Work out the finished part from the listing and answer in its coordinate system (mm). Round coordinates to 2 decimals unless told otherwise and drop trailing zeros. Loops run counter-clockwise (first coordinate to the right, second up) from the corner with the lowest first, then second, coordinate; pieces in that order, holes last. Notation, with made-up numbers: (34, -39.75) - (92, -39.75) arc R18 ccw to (92, -33.75) - close; hole circle Ø4 at (-26.5, 20.25). An arc over 180 degrees is marked (long way). Return JSON: item names as keys, results as strings.
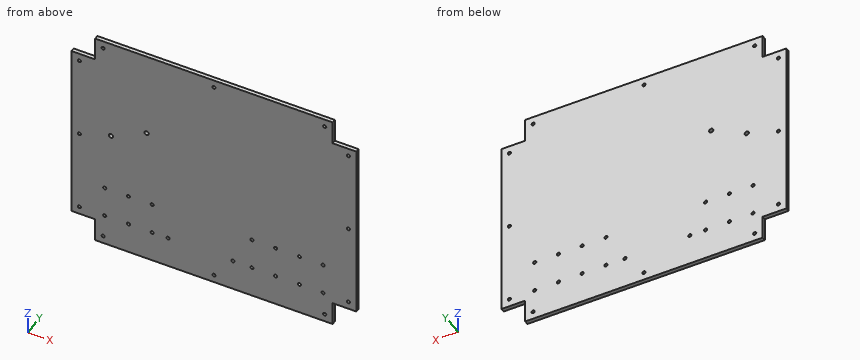
from build123d import *

# Parameters (mm, degrees)
SKETCH1_W           = 457.2
SKETCH1_H           = 368.3
SKETCH1_R           = 2.5527
BOSS_EXTRUDE1_DEPTH = 6.35
CUT_EXTRUDE1_REACH  = 589.126
SKETCH2_W           = 38.1
SKETCH2_H           = 38.1
CUT_EXTRUDE2_REACH  = 589.126
SKETCH3_R           = 2.5527
CUT_EXTRUDE3_REACH  = 589.126
SKETCH5_R           = 3.429


with BuildPart() as part:
    # Sketch1 → Boss-Extrude1 (new body)
    with BuildSketch(Plane(origin=(0, 0, 0), x_dir=(1, 0, 0), z_dir=(0, 1, 0))):
        with Locations((228.6, 184.15)):
            Rectangle(SKETCH1_W, SKETCH1_H)
        with Locations(Location((50.8, 355.6, 0), (0, 0, 270))):
            Circle(SKETCH1_R, mode=Mode.SUBTRACT)
        with Locations(Location((406.4, 355.6, 0), (0, 0, 270))):
            Circle(SKETCH1_R, mode=Mode.SUBTRACT)
        with Locations(Location((406.4, 12.7, 0), (0, 0, 270))):
            Circle(SKETCH1_R, mode=Mode.SUBTRACT)
        with Locations(Location((50.8, 12.7, 0), (0, 0, 270))):
            Circle(SKETCH1_R, mode=Mode.SUBTRACT)
        with Locations(Location((228.6, 12.7, 0), (0, 0, 270))):
            Circle(SKETCH1_R, mode=Mode.SUBTRACT)
        with Locations(Location((228.6, 355.6, 0), (0, 0, 270))):
            Circle(SKETCH1_R, mode=Mode.SUBTRACT)
        with Locations(Location((12.7, 184.15, 0), (0, 0, 270))):
            Circle(SKETCH1_R, mode=Mode.SUBTRACT)
        with Locations(Location((444.5, 184.15, 0), (0, 0, 270))):
            Circle(SKETCH1_R, mode=Mode.SUBTRACT)
        with Locations(Location((12.7, 50.8, 0), (0, 0, 270))):
            Circle(SKETCH1_R, mode=Mode.SUBTRACT)
        with Locations(Location((444.5, 50.8, 0), (0, 0, 270))):
            Circle(SKETCH1_R, mode=Mode.SUBTRACT)
        with Locations(Location((444.5, 317.5, 0), (0, 0, 270))):
            Circle(SKETCH1_R, mode=Mode.SUBTRACT)
        with Locations(Location((12.7, 317.5, 0), (0, 0, 270))):
            Circle(SKETCH1_R, mode=Mode.SUBTRACT)
    extrude(amount=BOSS_EXTRUDE1_DEPTH)

    # Sketch2 → Cut-Extrude1 (cut, up to next)
    with BuildSketch(Plane(origin=(0, 6.35, 0), x_dir=(1, 0, 0), z_dir=(0, 1, 0)), mode=Mode.PRIVATE) as cut_extrude1_sk1:
        with Locations((19.05, 19.05)):
            Rectangle(SKETCH2_W, SKETCH2_H)
    cut_extrude1_tool1 = extrude(cut_extrude1_sk1.sketch, amount=-CUT_EXTRUDE1_REACH, mode=Mode.PRIVATE) & part.part
    # Sketch2 → Cut-Extrude1 (cut, up to next)
    with BuildSketch(Plane(origin=(0, 6.35, 0), x_dir=(1, 0, 0), z_dir=(0, 1, 0)), mode=Mode.PRIVATE) as cut_extrude1_sk2:
        with Locations((19.05, 349.25)):
            Rectangle(SKETCH2_W, SKETCH2_H)
    cut_extrude1_tool2 = extrude(cut_extrude1_sk2.sketch, amount=-CUT_EXTRUDE1_REACH, mode=Mode.PRIVATE) & part.part
    # Sketch2 → Cut-Extrude1 (cut, up to next)
    with BuildSketch(Plane(origin=(0, 6.35, 0), x_dir=(1, 0, 0), z_dir=(0, 1, 0)), mode=Mode.PRIVATE) as cut_extrude1_sk3:
        with Locations((438.15, 349.25)):
            Rectangle(SKETCH2_W, SKETCH2_H)
    cut_extrude1_tool3 = extrude(cut_extrude1_sk3.sketch, amount=-CUT_EXTRUDE1_REACH, mode=Mode.PRIVATE) & part.part
    # Sketch2 → Cut-Extrude1 (cut, up to next)
    with BuildSketch(Plane(origin=(0, 6.35, 0), x_dir=(1, 0, 0), z_dir=(0, 1, 0)), mode=Mode.PRIVATE) as cut_extrude1_sk4:
        with Locations((438.15, 19.05)):
            Rectangle(SKETCH2_W, SKETCH2_H)
    cut_extrude1_tool4 = extrude(cut_extrude1_sk4.sketch, amount=-CUT_EXTRUDE1_REACH, mode=Mode.PRIVATE) & part.part
    add(cut_extrude1_tool1.solids().sort_by_distance((19.05, 6.35, -19.05))[0], mode=Mode.SUBTRACT)
    add(cut_extrude1_tool2.solids().sort_by_distance((19.05, 6.35, -349.25))[0], mode=Mode.SUBTRACT)
    add(cut_extrude1_tool3.solids().sort_by_distance((438.15, 6.35, -349.25))[0], mode=Mode.SUBTRACT)
    add(cut_extrude1_tool4.solids().sort_by_distance((438.15, 6.35, -19.05))[0], mode=Mode.SUBTRACT)

    # Sketch3 → Cut-Extrude2 (cut, up to next)
    with BuildSketch(Plane(origin=(0, 6.35, 0), x_dir=(1, 0, 0), z_dir=(0, 1, 0)), mode=Mode.PRIVATE) as cut_extrude2_sk1:
        with Locations(Location((53.34, 266.7, 0), (0, 0, 270))):
            Circle(SKETCH3_R)
    cut_extrude2_tool1 = extrude(cut_extrude2_sk1.sketch, amount=-CUT_EXTRUDE2_REACH, mode=Mode.PRIVATE) & part.part
    # Sketch3 → Cut-Extrude2 (cut, up to next)
    with BuildSketch(Plane(origin=(0, 6.35, 0), x_dir=(1, 0, 0), z_dir=(0, 1, 0)), mode=Mode.PRIVATE) as cut_extrude2_sk2:
        with Locations(Location((53.34, 317.5, 0), (0, 0, 270))):
            Circle(SKETCH3_R)
    cut_extrude2_tool2 = extrude(cut_extrude2_sk2.sketch, amount=-CUT_EXTRUDE2_REACH, mode=Mode.PRIVATE) & part.part
    # Sketch3 → Cut-Extrude2 (cut, up to next)
    with BuildSketch(Plane(origin=(0, 6.35, 0), x_dir=(1, 0, 0), z_dir=(0, 1, 0)), mode=Mode.PRIVATE) as cut_extrude2_sk3:
        with Locations(Location((91.44, 266.7, 0), (0, 0, 270))):
            Circle(SKETCH3_R)
    cut_extrude2_tool3 = extrude(cut_extrude2_sk3.sketch, amount=-CUT_EXTRUDE2_REACH, mode=Mode.PRIVATE) & part.part
    # Sketch3 → Cut-Extrude2 (cut, up to next)
    with BuildSketch(Plane(origin=(0, 6.35, 0), x_dir=(1, 0, 0), z_dir=(0, 1, 0)), mode=Mode.PRIVATE) as cut_extrude2_sk4:
        with Locations(Location((91.44, 317.5, 0), (0, 0, 270))):
            Circle(SKETCH3_R)
    cut_extrude2_tool4 = extrude(cut_extrude2_sk4.sketch, amount=-CUT_EXTRUDE2_REACH, mode=Mode.PRIVATE) & part.part
    # Sketch3 → Cut-Extrude2 (cut, up to next)
    with BuildSketch(Plane(origin=(0, 6.35, 0), x_dir=(1, 0, 0), z_dir=(0, 1, 0)), mode=Mode.PRIVATE) as cut_extrude2_sk5:
        with Locations(Location((129.54, 266.7, 0), (0, 0, 270))):
            Circle(SKETCH3_R)
    cut_extrude2_tool5 = extrude(cut_extrude2_sk5.sketch, amount=-CUT_EXTRUDE2_REACH, mode=Mode.PRIVATE) & part.part
    # Sketch3 → Cut-Extrude2 (cut, up to next)
    with BuildSketch(Plane(origin=(0, 6.35, 0), x_dir=(1, 0, 0), z_dir=(0, 1, 0)), mode=Mode.PRIVATE) as cut_extrude2_sk6:
        with Locations(Location((129.54, 317.5, 0), (0, 0, 270))):
            Circle(SKETCH3_R)
    cut_extrude2_tool6 = extrude(cut_extrude2_sk6.sketch, amount=-CUT_EXTRUDE2_REACH, mode=Mode.PRIVATE) & part.part
    # Sketch3 → Cut-Extrude2 (cut, up to next)
    with BuildSketch(Plane(origin=(0, 6.35, 0), x_dir=(1, 0, 0), z_dir=(0, 1, 0)), mode=Mode.PRIVATE) as cut_extrude2_sk7:
        with Locations(Location((289.56, 266.7, 0), (0, 0, 270))):
            Circle(SKETCH3_R)
    cut_extrude2_tool7 = extrude(cut_extrude2_sk7.sketch, amount=-CUT_EXTRUDE2_REACH, mode=Mode.PRIVATE) & part.part
    # Sketch3 → Cut-Extrude2 (cut, up to next)
    with BuildSketch(Plane(origin=(0, 6.35, 0), x_dir=(1, 0, 0), z_dir=(0, 1, 0)), mode=Mode.PRIVATE) as cut_extrude2_sk8:
        with Locations(Location((289.56, 317.5, 0), (0, 0, 270))):
            Circle(SKETCH3_R)
    cut_extrude2_tool8 = extrude(cut_extrude2_sk8.sketch, amount=-CUT_EXTRUDE2_REACH, mode=Mode.PRIVATE) & part.part
    # Sketch3 → Cut-Extrude2 (cut, up to next)
    with BuildSketch(Plane(origin=(0, 6.35, 0), x_dir=(1, 0, 0), z_dir=(0, 1, 0)), mode=Mode.PRIVATE) as cut_extrude2_sk9:
        with Locations(Location((403.86, 266.7, 0), (0, 0, 270))):
            Circle(SKETCH3_R)
    cut_extrude2_tool9 = extrude(cut_extrude2_sk9.sketch, amount=-CUT_EXTRUDE2_REACH, mode=Mode.PRIVATE) & part.part
    # Sketch3 → Cut-Extrude2 (cut, up to next)
    with BuildSketch(Plane(origin=(0, 6.35, 0), x_dir=(1, 0, 0), z_dir=(0, 1, 0)), mode=Mode.PRIVATE) as cut_extrude2_sk10:
        with Locations(Location((403.86, 317.5, 0), (0, 0, 270))):
            Circle(SKETCH3_R)
    cut_extrude2_tool10 = extrude(cut_extrude2_sk10.sketch, amount=-CUT_EXTRUDE2_REACH, mode=Mode.PRIVATE) & part.part
    # Sketch3 → Cut-Extrude2 (cut, up to next)
    with BuildSketch(Plane(origin=(0, 6.35, 0), x_dir=(1, 0, 0), z_dir=(0, 1, 0)), mode=Mode.PRIVATE) as cut_extrude2_sk11:
        with Locations(Location((365.76, 266.7, 0), (0, 0, 270))):
            Circle(SKETCH3_R)
    cut_extrude2_tool11 = extrude(cut_extrude2_sk11.sketch, amount=-CUT_EXTRUDE2_REACH, mode=Mode.PRIVATE) & part.part
    # Sketch3 → Cut-Extrude2 (cut, up to next)
    with BuildSketch(Plane(origin=(0, 6.35, 0), x_dir=(1, 0, 0), z_dir=(0, 1, 0)), mode=Mode.PRIVATE) as cut_extrude2_sk12:
        with Locations(Location((365.76, 317.5, 0), (0, 0, 270))):
            Circle(SKETCH3_R)
    cut_extrude2_tool12 = extrude(cut_extrude2_sk12.sketch, amount=-CUT_EXTRUDE2_REACH, mode=Mode.PRIVATE) & part.part
    # Sketch3 → Cut-Extrude2 (cut, up to next)
    with BuildSketch(Plane(origin=(0, 6.35, 0), x_dir=(1, 0, 0), z_dir=(0, 1, 0)), mode=Mode.PRIVATE) as cut_extrude2_sk13:
        with Locations(Location((327.66, 266.7, 0), (0, 0, 270))):
            Circle(SKETCH3_R)
    cut_extrude2_tool13 = extrude(cut_extrude2_sk13.sketch, amount=-CUT_EXTRUDE2_REACH, mode=Mode.PRIVATE) & part.part
    # Sketch3 → Cut-Extrude2 (cut, up to next)
    with BuildSketch(Plane(origin=(0, 6.35, 0), x_dir=(1, 0, 0), z_dir=(0, 1, 0)), mode=Mode.PRIVATE) as cut_extrude2_sk14:
        with Locations(Location((327.66, 317.5, 0), (0, 0, 270))):
            Circle(SKETCH3_R)
    cut_extrude2_tool14 = extrude(cut_extrude2_sk14.sketch, amount=-CUT_EXTRUDE2_REACH, mode=Mode.PRIVATE) & part.part
    # Sketch3 → Cut-Extrude2 (cut, up to next)
    with BuildSketch(Plane(origin=(0, 6.35, 0), x_dir=(1, 0, 0), z_dir=(0, 1, 0)), mode=Mode.PRIVATE) as cut_extrude2_sk15:
        with Locations(Location((259.08, 317.5, 0), (0, 0, 270))):
            Circle(SKETCH3_R)
    cut_extrude2_tool15 = extrude(cut_extrude2_sk15.sketch, amount=-CUT_EXTRUDE2_REACH, mode=Mode.PRIVATE) & part.part
    # Sketch3 → Cut-Extrude2 (cut, up to next)
    with BuildSketch(Plane(origin=(0, 6.35, 0), x_dir=(1, 0, 0), z_dir=(0, 1, 0)), mode=Mode.PRIVATE) as cut_extrude2_sk16:
        with Locations(Location((154.94, 317.5, 0), (0, 0, 270))):
            Circle(SKETCH3_R)
    cut_extrude2_tool16 = extrude(cut_extrude2_sk16.sketch, amount=-CUT_EXTRUDE2_REACH, mode=Mode.PRIVATE) & part.part
    add(cut_extrude2_tool1.solids().sort_by_distance((53.34, 6.35, -266.7))[0], mode=Mode.SUBTRACT)
    add(cut_extrude2_tool2.solids().sort_by_distance((53.34, 6.35, -317.5))[0], mode=Mode.SUBTRACT)
    add(cut_extrude2_tool3.solids().sort_by_distance((91.44, 6.35, -266.7))[0], mode=Mode.SUBTRACT)
    add(cut_extrude2_tool4.solids().sort_by_distance((91.44, 6.35, -317.5))[0], mode=Mode.SUBTRACT)
    add(cut_extrude2_tool5.solids().sort_by_distance((129.54, 6.35, -266.7))[0], mode=Mode.SUBTRACT)
    add(cut_extrude2_tool6.solids().sort_by_distance((129.54, 6.35, -317.5))[0], mode=Mode.SUBTRACT)
    add(cut_extrude2_tool7.solids().sort_by_distance((289.56, 6.35, -266.7))[0], mode=Mode.SUBTRACT)
    add(cut_extrude2_tool8.solids().sort_by_distance((289.56, 6.35, -317.5))[0], mode=Mode.SUBTRACT)
    add(cut_extrude2_tool9.solids().sort_by_distance((403.86, 6.35, -266.7))[0], mode=Mode.SUBTRACT)
    add(cut_extrude2_tool10.solids().sort_by_distance((403.86, 6.35, -317.5))[0], mode=Mode.SUBTRACT)
    add(cut_extrude2_tool11.solids().sort_by_distance((365.76, 6.35, -266.7))[0], mode=Mode.SUBTRACT)
    add(cut_extrude2_tool12.solids().sort_by_distance((365.76, 6.35, -317.5))[0], mode=Mode.SUBTRACT)
    add(cut_extrude2_tool13.solids().sort_by_distance((327.66, 6.35, -266.7))[0], mode=Mode.SUBTRACT)
    add(cut_extrude2_tool14.solids().sort_by_distance((327.66, 6.35, -317.5))[0], mode=Mode.SUBTRACT)
    add(cut_extrude2_tool15.solids().sort_by_distance((259.08, 6.35, -317.5))[0], mode=Mode.SUBTRACT)
    add(cut_extrude2_tool16.solids().sort_by_distance((154.94, 6.35, -317.5))[0], mode=Mode.SUBTRACT)

    # Sketch5 → Cut-Extrude3 (cut, up to next)
    with BuildSketch(Plane.XZ, mode=Mode.PRIVATE) as cut_extrude3_sk1:
        with Locations(Location((63.5, -167.64, 0), (0, 0, 270))):
            Circle(SKETCH5_R)
    cut_extrude3_tool1 = extrude(cut_extrude3_sk1.sketch, amount=-CUT_EXTRUDE3_REACH, mode=Mode.PRIVATE) & part.part
    # Sketch5 → Cut-Extrude3 (cut, up to next)
    with BuildSketch(Plane.XZ, mode=Mode.PRIVATE) as cut_extrude3_sk2:
        with Locations(Location((120.65, -139.7, 0), (0, 0, 270))):
            Circle(SKETCH5_R)
    cut_extrude3_tool2 = extrude(cut_extrude3_sk2.sketch, amount=-CUT_EXTRUDE3_REACH, mode=Mode.PRIVATE) & part.part
    add(cut_extrude3_tool1.solids().sort_by_distance((63.5, 0, -167.64))[0], mode=Mode.SUBTRACT)
    add(cut_extrude3_tool2.solids().sort_by_distance((120.65, 0, -139.7))[0], mode=Mode.SUBTRACT)


solid = part.part
1) Section B-B (z = -31) is taken. Give the vertices of the cut face in (x, y), and give its area (3 significant figures).
Verdict:
{"outline": "(38.1, 0) - (419.1, 0) - (419.1, 6.35) - (38.1, 6.35) - close", "area": "2,420 mm2"}
2) Section A-A (y = 4.5) is taken. Count the separate pieces of the cut face and the enclosed holes in it, and give its area (3 significant figures).
Verdict:
{"separate pieces": "1", "enclosed holes": "30", "area": "162,000 mm2"}
3) Flat-ended cylindrical pins translate along their axes: pin 1 (1.9 mm diameter, centred on x = 444.5, y = 4, fed in from +Z); pin 2 (1.9 mm diameter, centred on y = 3, z = -18, fed in from +X). Find the tip coordinate at first contact, or state that the pin passes through.
Verdict:
{"pin 1": "stops at z = -38.1", "pin 2": "stops at x = 419.1"}
4) Find the intervals of material crossed by L1, parallel to X at y = 4.5, z = -12.7; L2, parallel to Z at x = 365.76, y = 1.5; L3, parallel to X at y = 3, z = -140, in increasing order.
Verdict:
{"L1": "x = 38.1 to 48.25, 53.35 to 226.05, 231.15 to 403.85, 408.95 to 419.1", "L2": "z = -368.3 to -320.05, -314.95 to -269.25, -264.15 to 0", "L3": "x = 0 to 117.23, 124.07 to 457.2"}
